from build123d import *

# Parameters (mm, degrees)
SKETCH1_R           = 2
SKETCH1_W           = 12.7
SKETCH1_H           = 50.8
BOSS_EXTRUDE3_DEPTH = 6.35


with BuildPart() as part:
    # Sketch1 → Boss-Extrude3 (new body)
    with BuildSketch(Plane(origin=(0, 0, 0), x_dir=(1, 0, 0), z_dir=(0, 1, 0))):
        with BuildLine():
            ThreePointArc((34.194833578, -66.63583839), (33.11372382, -66.748004461), (32.240681933, -66.10056535))
            ThreePointArc((32.240681933, -66.10056535), (0, -48.302004425), (-32.240681933, -66.10056535))
            ThreePointArc((-32.240681933, -66.10056535), (-33.11372382, -66.748004461), (-34.194833578, -66.63583839))
            ThreePointArc((-34.194833578, -66.63583839), (0, 74.897407173), (34.194833578, -66.63583839))
        make_face()
        with Locations((0, 53.061187965)):
            Circle(SKETCH1_R, mode=Mode.SUBTRACT)
        with Locations((18.178952795, 24.310551096)):
            Circle(SKETCH1_R, mode=Mode.SUBTRACT)
        with Locations((46.663733983, 40.081231883)):
            Circle(SKETCH1_R, mode=Mode.SUBTRACT)
        with Locations((46.663733983, -40.081231883)):
            Circle(SKETCH1_R, mode=Mode.SUBTRACT)
        with Locations((-46.663733983, -40.081231883)):
            Circle(SKETCH1_R, mode=Mode.SUBTRACT)
        with Locations((-18.178952795, 24.310551096)):
            Circle(SKETCH1_R, mode=Mode.SUBTRACT)
        with Locations((-46.663733983, 40.081231883)):
            Circle(SKETCH1_R, mode=Mode.SUBTRACT)
        with Locations((61.164123727, 0)):
            Rectangle(SKETCH1_W, SKETCH1_H, mode=Mode.SUBTRACT)
        with Locations((-61.164123727, 0)):
            Rectangle(SKETCH1_W, SKETCH1_H, mode=Mode.SUBTRACT)
        with BuildLine():
            ThreePointArc((-5.853899988, 60.78531778), (0.003726822, 57.376699875), (5.857575472, 60.791802193))
            ThreePointArc((5.857575472, 60.791802193), (10.16, 64.107698843), (5.857575472, 67.423595493))
            ThreePointArc((5.857575472, 67.423595493), (0.003726822, 70.838697812), (-5.853899988, 67.430079907))
            ThreePointArc((-5.853899988, 67.430079907), (-10.167207264, 64.107698843), (-5.853899988, 60.78531778))
        make_face(mode=Mode.SUBTRACT)
    extrude(amount=BOSS_EXTRUDE3_DEPTH)


solid = part.part
Check sheet for the modelled part. Datum: model origin and axes. Units: mm. A direction names the side the tool comes from. Round coordinates to 2 decimals unless told otherwise and drop trailing zeros. Order: outer loops, then holes, each group sorted by start corner. A loop starts at its lowest first (then second) coordinate and runs counter-clockwise, first axis right, second up.
(1) Go/stop test with flat-tipped pins: P1, Ø2, axis at y = 5, z = -44, coming from the -X side; P2, Ø3, axis at x = -64, y = 4.5, coming from the +Z side; P3, Ø3, axis at x = -61.5, y = 3, coming from the -Z side. Record where each tip stops, or that it passes through.
(2) Cross-section at D-D, the plane z = -64.5. Enter the section's corners in (x, y), and give its area (3 significant figures).
(3) Draft check along X on faces 3 (the flat face through (1, 6.35, -5)), 4 (the cylindrical face through (10.16, 3.13, -64.02)). Enter one of: pulls with the +X half, pulls with the -X half, needs draft (parallel to the pull), parting line crosses it, or undercut.
(4) Scan lines: probe 1 along X at (y, z) = (2, 9); probe 2 along X at (y, z) = (2.25, 13); probe 3 along Z at (x, y) = (-45, 5.5). Record each from-to range of solid material in increasing order.
(5) Cross-section at B-B, the plane x = 0. Enter the section's corners in (y, z), and give its area (3 significant figures).
(6) Cross-section at C-C, the plane x = 63.5. Enter the section's corners in (y, z), and give its area (3 significant figures).
(7) Cross-section at A-A, the plane z = 0. Enter the section's corners in (x, y).
(8) Access from +Z, -Z, +X, -X, +Y, -Y to the whole of each face (thin tool, end or side, straight path). Record for faces 1 (the flat face through (67.514, 3, 0)), 2 (the cylindrical face through (0.538, 3.131, 48.306)).
Check sheet entries:
1. P1: stops at x = -61.32
1. P2: stops at z = 41.27
1. P3: stops at z = -44.83
2. outline: (-38.07, 0) - (-10.14, 0) - (-10.14, 6.35) - (-38.07, 6.35) - close; (10.14, 0) - (38.07, 0) - (38.07, 6.35) - (10.14, 6.35) - close
2. area: 355 mm2
3. face 3: needs draft
3. face 4: undercut
4. probe 1: x = -74.35 to -67.51, -54.81 to 54.81, 67.51 to 74.35
4. probe 2: x = -73.76 to -67.51, -54.81 to 54.81, 67.51 to 73.76
4. probe 3: z = -59.87 to -41.19, -38.97 to 38.97, 41.19 to 59.87
5. outline: (0, -74.9) - (6.35, -74.9) - (6.35, -70.84) - (0, -70.84) - close; (0, -57.38) - (6.35, -57.38) - (6.35, -55.06) - (0, -55.06) - close; (0, -51.06) - (6.35, -51.06) - (6.35, 48.3) - (0, 48.3) - close
5. area: 671 mm2
6. outline: (0, -39.72) - (6.35, -39.72) - (6.35, -25.4) - (0, -25.4) - close; (0, 25.4) - (6.35, 25.4) - (6.35, 39.72) - (0, 39.72) - close
6. area: 182 mm2
7. outline: (-74.9, 0) - (-67.51, 0) - (-67.51, 6.35) - (-74.9, 6.35) - close; (-54.81, 0) - (54.81, 0) - (54.81, 6.35) - (-54.81, 6.35) - close; (67.51, 0) - (74.9, 0) - (74.9, 6.35) - (67.51, 6.35) - close
8. face 1: +Y, -Y
8. face 2: +Z, +Y, -Y
